The figure shows three views and two pictorial views of one solid part (mm, origin at its lowest corner). Answer the questions. Coordinates: 2 decimals unless noted, no trailing zeros. Order: outer loops, then holes, each group sorted by start corner. A loop starts at its lowest first (then second) coordinate and runs counter-clockwise, first axis right, second up. Notation, with made-up numbers: M 62.5,19.5 L 106.5,19.5 A7 ccw 106.5,30.5 Z; hole C 73.25,-39 d8. An arc over 180 degrees is marked long. Answer in a Markdown table with one row per item. Add a question column.
Item 1: The part is cut by section A-A (x = 22.55). Write down the section's boundary in (y, z).
Item 2: Consider line 1 (Z direction, x = 22.55, y = 1.2); line 2 (Z direction, x = 20.5, y = 1.45); line 3 (Z direction, x = 29.5, y = 2). Determine where each line is inside the solid, lowest interval first. Write a range as from..to.
Item 3: A flat-ended cylindrical pin translates along its axis: pin 1 Ø3.5 at (x, z) = (22.55, 53.05) entering from -Y. Find the tip coordinate at first contact, or state that the pin passes through.
Item 4: The part is cut by section C-C (y = 0.7). Write down the section's boundary in (x, z), then the cut area to 3 significant figures.
Item 5: The part is cut by section B-B (z = 30.5). Write down the section's boundary in (x, y), then the cut area to 3 significant figures.
Item 6: The part is cut by section D-D (x = 13.5). Write down the section's boundary in (y, z).
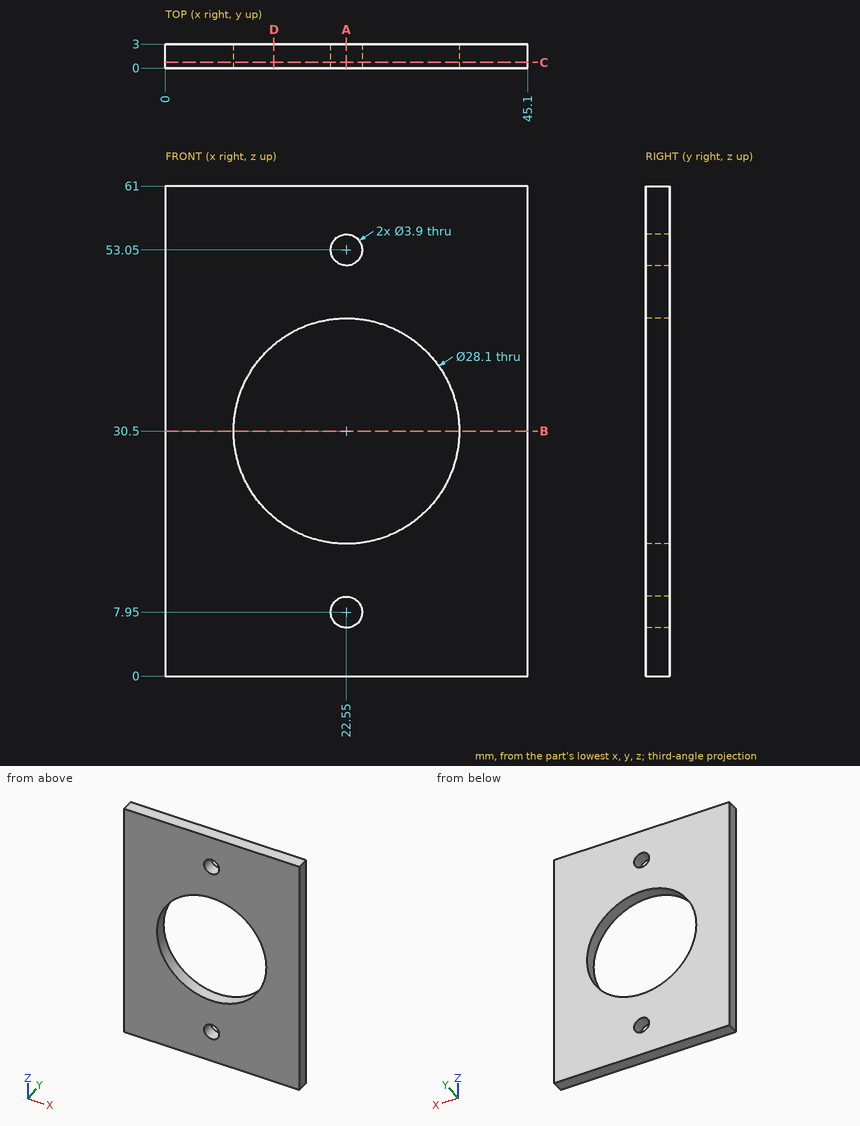
Reply:
| question | item | result |
|---|---|---|
| 1 | outline | M 0,0 L 3,0 L 3,6 L 0,6 Z; M 0,9.9 L 3,9.9 L 3,16.45 L 0,16.45 Z; M 0,44.55 L 3,44.55 L 3,51.1 L 0,51.1 Z; M 0,55 L 3,55 L 3,61 L 0,61 Z |
| 2 | line 1 | z = 0..6, 9.9..16.45, 44.55..51.1, 55..61 |
| 2 | line 2 | z = 0..16.6, 44.4..61 |
| 2 | line 3 | z = 0..18.29, 42.71..61 |
| 3 | pin 1 | passes through |
| 4 | outline | M 0,0 L 45.1,0 L 45.1,61 L 0,61 Z; hole C 22.55,30.5 d28.1; hole C 22.55,7.95 d3.9; hole C 22.55,53.05 d3.9 |
| 4 | area | 2,110 mm2 |
| 5 | outline | M 0,0 L 8.5,0 L 8.5,3 L 0,3 Z; M 36.6,0 L 45.1,0 L 45.1,3 L 36.6,3 Z |
| 5 | area | 51.0 mm2 |
| 6 | outline | M 0,0 L 3,0 L 3,19.75 L 0,19.75 Z; M 0,41.25 L 3,41.25 L 3,61 L 0,61 Z |
